from build123d import *

# Parameters (mm, degrees)
SKETCH_1_R           = 12.5
EXTRUDE_2_DEPTH      = 235.43
SKETCH_2_R           = 9
CUT_EXTRUDE_1_DEPTH  = 235.43
EXTRUDE_START        = 15.57
SKETCH_3_R           = 12.5
EXTRUDE_3_DEPTH      = 15.57
SKETCH_4_R           = 9
CUT_EXTRUDE_2_DEPTH  = 20
EXTRUDE_START_2      = 9.93
SKETCH_5_R           = 12.5
EXTRUDE_4_DEPTH      = 9.93
SKETCH_6_R           = 9
CUT_EXTRUDE_3_DEPTH  = 10
SKETCH_7_R           = 26.85848727
CUT_EXTRUDE_4_DEPTH  = 14.93
SKETCH_8_R           = 12.5
EXTRUDE_5_DEPTH      = 9.93
SKETCH_9_R           = 9
CUT_EXTRUDE_5_DEPTH  = 10
SKETCH_10_R          = 37.193394561
CUT_EXTRUDE_6_DEPTH  = 0.22
SKETCH_11_R          = 43.187188263
CUT_EXTRUDE_7_DEPTH  = 0.71
SKETCH_12_R          = 12.5
EXTRUDE_6_DEPTH      = 15
CUT_EXTRUDE_START    = -15
SKETCH_13_R          = 9
CUT_EXTRUDE_8_DEPTH  = 15
SKETCH_14_R          = 46.427055536
CUT_EXTRUDE_9_DEPTH  = 85
SKETCH_15_R          = 11
CUT_EXTRUDE_10_DEPTH = 324


with BuildPart() as part:
    # 草图1 → 凸台-拉伸2 (new body)
    with BuildSketch(Plane.XY):
        Circle(SKETCH_1_R)
    extrude(amount=EXTRUDE_2_DEPTH)

    # 草图2 → 切除-拉伸1 (cut)
    with BuildSketch(Plane(origin=(0, 0, 0), x_dir=(-1, 0, 0), z_dir=(0, 0, -1))):
        Circle(SKETCH_2_R)
    extrude(amount=-CUT_EXTRUDE_1_DEPTH, mode=Mode.SUBTRACT)

    # 草图3 → 凸台-拉伸3 (add)
    with BuildSketch(Plane(origin=(0, 0, 0), x_dir=(-1, 0, 0), z_dir=(0, 0, -1)).offset(EXTRUDE_START)):
        Circle(SKETCH_3_R)
    extrude(amount=-EXTRUDE_3_DEPTH)

    # 草图4 → 切除-拉伸2 (cut)
    with BuildSketch(Plane(origin=(0, 0, -15.57), x_dir=(-1, 0, 0), z_dir=(0, 0, -1))):
        Circle(SKETCH_4_R)
    extrude(amount=-CUT_EXTRUDE_2_DEPTH, mode=Mode.SUBTRACT)

    # 草图5 → 凸台-拉伸4 (add)
    with BuildSketch(Plane(origin=(0, 0, -15.57), x_dir=(-1, 0, 0), z_dir=(0, 0, -1)).offset(EXTRUDE_START_2)):
        Circle(SKETCH_5_R)
    extrude(amount=-EXTRUDE_4_DEPTH)

    # 草图6 → 切除-拉伸3 (cut)
    with BuildSketch(Plane(origin=(0, 0, -25.5), x_dir=(-1, 0, 0), z_dir=(0, 0, -1))):
        Circle(SKETCH_6_R)
    extrude(amount=-CUT_EXTRUDE_3_DEPTH, mode=Mode.SUBTRACT)

    # 草图7 → 切除-拉伸4 (cut)
    with BuildSketch(Plane(origin=(0, 0, -25.5), x_dir=(-1, 0, 0), z_dir=(0, 0, -1))):
        Circle(SKETCH_7_R)
    extrude(amount=-CUT_EXTRUDE_4_DEPTH, mode=Mode.SUBTRACT)

    # 草图8 → 凸台-拉伸5 (add)
    with BuildSketch(Plane(origin=(0, 0, -10.57), x_dir=(-1, 0, 0), z_dir=(0, 0, -1)).offset(EXTRUDE_START_2)):
        Circle(SKETCH_8_R)
    extrude(amount=-EXTRUDE_5_DEPTH)

    # 草图9 → 切除-拉伸5 (cut)
    with BuildSketch(Plane(origin=(0, 0, -20.5), x_dir=(-1, 0, 0), z_dir=(0, 0, -1))):
        Circle(SKETCH_9_R)
    extrude(amount=-CUT_EXTRUDE_5_DEPTH, mode=Mode.SUBTRACT)

    # 草图10 → 切除-拉伸6 (cut)
    with BuildSketch(Plane(origin=(0, 0, -20.5), x_dir=(-1, 0, 0), z_dir=(0, 0, -1))):
        with Locations((7.201744855, 7.507888779)):
            Circle(SKETCH_10_R)
    extrude(amount=-CUT_EXTRUDE_6_DEPTH, mode=Mode.SUBTRACT)

    # 草图11 → 切除-拉伸7 (cut)
    with BuildSketch(Plane(origin=(0, 0, -20.28), x_dir=(-1, 0, 0), z_dir=(0, 0, -1))):
        with Locations((-1.225460352, 2.329416421)):
            Circle(SKETCH_11_R)
    extrude(amount=-CUT_EXTRUDE_7_DEPTH, mode=Mode.SUBTRACT)

    # 草图12 → 凸台-拉伸6 (add)
    with BuildSketch(Plane.XY.offset(235.43)):
        with Locations(Location((0, 0, 0), (0, 0, 180))):
            Circle(SKETCH_12_R)
    extrude(amount=EXTRUDE_6_DEPTH)

    # 草图13 → 切除-拉伸8 (cut)
    with BuildSketch(Plane.XY.offset(250.43).offset(CUT_EXTRUDE_START)):
        with Locations(Location((0, 0, 0), (0, 0, 180))):
            Circle(SKETCH_13_R)
    extrude(amount=CUT_EXTRUDE_8_DEPTH, mode=Mode.SUBTRACT)

    # 草图14 → 切除-拉伸9 (cut)
    with BuildSketch(Plane.XY.offset(250.43)):
        with Locations((-6.064552421, 3.817147789)):
            Circle(SKETCH_14_R)
    extrude(amount=-CUT_EXTRUDE_9_DEPTH, mode=Mode.SUBTRACT)

    # 草图15 → 切除-拉伸10 (cut)
    with BuildSketch(Plane.XY.offset(165.43)):
        Circle(SKETCH_15_R)
    extrude(amount=-CUT_EXTRUDE_10_DEPTH, mode=Mode.SUBTRACT)


solid = part.part
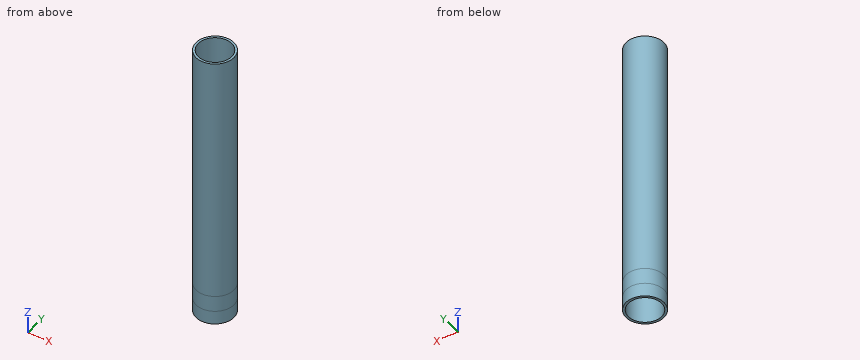
The listing builds one solid part. Answer for the finished solid, in the listing's coordinates (mm). Give positions to 0.01 mm unless a question says otherwise; leave off trailing zeros. Write each loop counter-clockwise with the first axis right and the second up, starting at its lowest first coordinate (ties: lowest second). Pieces come first, ordered by that corner, then holes. Notation, with made-up numbers: (1.5, 12.25) - (51.5, 12.25) arc R13 cw to (51.5, 16.25) - close; hole circle Ø9 at (-38, 33.5). An arc over 180 degrees is marked (long way). Use a Markdown table: item, result.
1. Find the intervals of material crossed by probe 1 along X at (y, z) = (0.5, 33.5); probe 2 along Y at (x, z) = (-8.25, 38), in increasing order. Write a range as from..to.
Values follow:
| item | result |
|---|---|
| probe 1 | x = -12.49..-10.99, 10.99..12.49 |
| probe 2 | y = -9.39..-7.28, 7.28..9.39 |
2. Section A-A on x = 0 is taken. Write down the section's boundary in (y, z), plus the area to 3 significant figures.
Values follow:
| item | result |
|---|---|
| outline | (-12.5, -19.57) - (-11, -19.57) - (-11, 165.43) - (-12.5, 165.43) - close; (11, -19.57) - (12.5, -19.57) - (12.5, 165.43) - (11, 165.43) - close |
| area | 555 mm² |
3. Section B-B on y = 2.75 is taken. Write down the section's boundary in (x, z).
Values follow:
| item | result |
|---|---|
| outline | (-12.19, -19.57) - (-10.65, -19.57) - (-10.65, 165.43) - (-12.19, 165.43) - close; (10.65, -19.57) - (12.19, -19.57) - (12.19, 165.43) - (10.65, 165.43) - close |
4. Each of these flat-tipped pins is pushed along its axis until it touches: P1, Ø3, axis at y = 3, z = 109, coming from the -X side; P2, Ø8, axis at x = 6, y = -0.5, coming from the -Z side; P3, Ø6, axis at x = -7, z = 145, coming from the -Y side; P4, Ø4, axis at x = -5, z = 0.5, coming from the +Y side. Where does it stop, or does it pass through?
Values follow:
| item | result |
|---|---|
| P1 | stops at x = -12.41 |
| P2 | passes through |
| P3 | stops at y = -11.84 |
| P4 | stops at y = 12.13 |
5. Section C-C on z = 72 is taken. Write down the section's boundary in (x, y).
Values follow:
| item | result |
|---|---|
| outline | circle Ø25 at (0, 0); hole circle Ø22 at (0, 0) |
